The figure shows three views and two pictorial views of one solid part (mm, origin at its lowest corner). Answer the questions. Coordinates: 2 decimals unless noted, no trailing zeros. Loops run counter-clockwise (first coordinate to the right, second up) from the corner with the lowest first, then second, coordinate; pieces in that order, holes last. Notation, with made-up numbers: (26.5, 77.5) -> (63.5, 77.5) arc R15 ccw to (63.5, 81.5) -> close; hole circle Ø8 at (53.25, -15.75). An arc over 180 degrees is marked (long way). Answer in a Markdown table with one row per item.
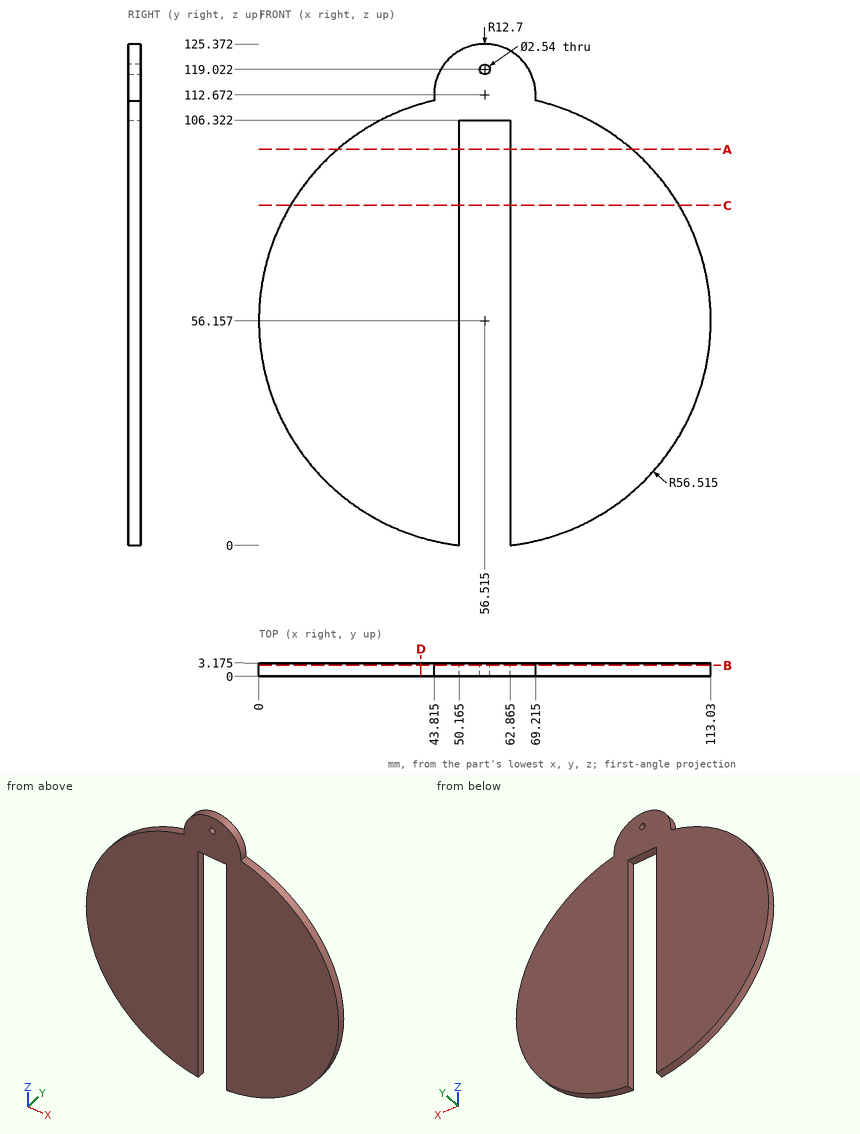
Item 1: Find the intervals of material crossed by probe 1 along X at (y, z) = (1.9, 58) (3 decimals); probe 2 along X at (y, z) = (2.5, 50) (1 decimal); probe 3 along Z at (x, y) = (55.5, 0.95) (1 decimal), in increasing order.
Findings below:
| item | result |
|---|---|
| probe 1 | x = 0.03 to 50.165, 62.865 to 113 |
| probe 2 | x = 0.3 to 50.2, 62.9 to 112.7 |
| probe 3 | z = 106.3 to 118.3, 119.8 to 125.3 |
Item 2: Flat-ended cylindrical pins translate along their axes: pin 1 Ø1 at (x, y) = (55.5, 2) entering from -Z; pin 2 Ø1.5 at (x, y) = (39.5, 2) entering from -Z; pin 3 Ø1.5 at (x, y) = (100.5, 1.5) entering from -Z. Find the tip coordinate at first contact, or state that the pin passes through.
Findings below:
| item | result |
|---|---|
| pin 1 | stops at z = 106.32 |
| pin 2 | stops at z = 2.03 |
| pin 3 | stops at z = 19.76 |
Item 3: A cutting plane is placed at A-A, the plane z = 99. Determine the outline of the cut face in (x, y) (3 decimals), plus the area to 3 significant figures.
Findings below:
| item | result |
|---|---|
| outline | (19.658, 0) -> (50.165, 0) -> (50.165, 3.175) -> (19.658, 3.175) -> close; (62.865, 0) -> (93.372, 0) -> (93.372, 3.175) -> (62.865, 3.175) -> close |
| area | 194 mm2 |
Item 4: A cutting plane is placed at C-C, the plane z = 85. Determine the outline of the cut face in (x, y) (1 decimal), plus the area to 3 significant figures.
Findings below:
| item | result |
|---|---|
| outline | (7.9, 0) -> (50.2, 0) -> (50.2, 3.2) -> (7.9, 3.2) -> close; (62.9, 0) -> (105.1, 0) -> (105.1, 3.2) -> (62.9, 3.2) -> close |
| area | 268 mm2 |
Item 5: A cutting plane is placed at B-B, the plane y = 2.65. Determine the outline of the cut face in (x, z) (1 decimal), plus the area to 3 significant figures.
Findings below:
| item | result |
|---|---|
| outline | (43.8, 111.2) arc R56.5 ccw to (50.2, 0) -> (50.2, 106.3) -> (62.9, 106.3) -> (62.9, 0) arc R56.5 ccw to (69.2, 111.2) -> (69.2, 112.7) arc R12.7 ccw to (43.8, 112.7) -> close; hole circle Ø2.5 at (56.5, 119) |
| area | 8,940 mm2 |
Item 6: A cutting plane is placed at D-D, the plane x = 40.5. Determine the outline of the cut face in (y, z) (1 decimal), plus the area to 3 significant figures.
Findings below:
| item | result |
|---|---|
| outline | (0, 2) -> (3.2, 2) -> (3.2, 110.4) -> (0, 110.4) -> close |
| area | 344 mm2 |
